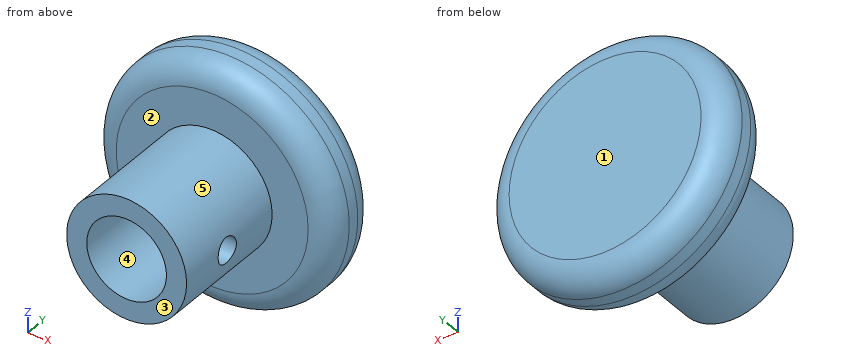
```python
from build123d import *

# Parameters (mm, degrees)
F0_R     = 6.35
F1_DEPTH = 19.05
F0_R_2   = 12.7
F2_DEPTH = 6.35
F4_D     = 8.4328
F4_DEPTH = 13.335
F4_TIP   = 2.5334687141
F6_R     = 2.54
F7_D     = 2.7051
F7_DEPTH = 7.62
F7_TIP   = 0.8126940303


with BuildPart() as f1:
    # F0 (on Front) → F1 (new body)
    with BuildSketch(Plane.XZ):
        Circle(F0_R)
    extrude(amount=F1_DEPTH)

    # F0 (on Front) → F2 (join)
    with BuildSketch(Plane.XZ):
        Circle(F0_R_2)
        Circle(F0_R, mode=Mode.SUBTRACT)
    extrude(amount=F2_DEPTH)

    # F4
    with Locations(Plane.XZ.offset(19.05)):
        with Locations((0, 0)):
            Hole(F4_D / 2, depth=F4_DEPTH)
            with Locations((0, 0, -(F4_DEPTH + F4_TIP / 2))):  # 118° drill point
                Cone(0, F4_D / 2, F4_TIP, mode=Mode.SUBTRACT)

    # F6
    f6_edges = [f1.edges().sort_by_distance(p)[0] for p in [
        (-12.7, -6.35, 0),
        (-12.7, 0, 0),
    ]]
    fillet(f6_edges, radius=F6_R)

    # F7 (one way)
    with BuildSketch(Plane(origin=(0, 0, 0), x_dir=(0, 1, 0), z_dir=(-1, 0, 0))):
        with Locations((-13.0086187273, 0)):
            Circle(F7_D / 2)
    extrude(amount=-F7_DEPTH, mode=Mode.SUBTRACT)
    with Locations(Plane(origin=(0, 0, 0), x_dir=(0, 1, 0), z_dir=(-1, 0, 0))):
        with Locations((-13.0086187273, 0)):
            with Locations((0, 0, -(F7_DEPTH + F7_TIP / 2))):  # 118° drill point
                Cone(0, F7_D / 2, F7_TIP, mode=Mode.SUBTRACT)


solid = f1.part
```
Could you check a few things on this model? Use its own coordinates, in mm. Face numbers are marked on the shaded views. A direction names the side the tool comes from. Round coordinates to 2 decimals unless told otherwise and drop trailing zeros. Write each loop counter-clockwise with the first axis right and the second up, starting at its lowest first coordinate (ties: lowest second). Pieces come first, ordered by that corner, then holes. Notation, with made-up numbers: M -33.75,55.5 L 20.25,55.5 A13 ccw 20.25,76.5 Z; hole C -3.5,22 d9. An arc over 180 degrees is marked long. Answer in a Markdown table with one row per item. Add a question column.
Q1. If we mould it in two halves opening along Z, with no side actions, what happens to the marked faces 3, 4 and 5? For each: +Z half, -Z half, draft (parallel to the pull), parting line (faces both ways), or undercut.
Q2. Imagine slicing it at A-A (y = -7.5). Please give me the cut outline in (x, z), then the cut area to 3 significant figures.
Q3. If I drill on line 1 (Z direction, x = 0, y = -11); line 2 (Z direction, x = 1.5, y = -13.5); line 3 (Y direction, x = 3, z = 7.25), over which ranges is the centre line in solid material (lowest first)? Write a range as from..to.
Q4. Will these pins go through, and if not, where does the flat tip stop? pin 1 Ø10 at (x, y) = (5, -12) entering from +Z; pin 2 Ø1 at (x, z) = (-7.5, 8.5) entering from +Y; pin 3 Ø11 at (x, z) = (0, 0) entering from +Y; pin 4 Ø8 at (x, z) = (10, 5) entering from -Y.
Q5. Imagine slicing it at B-B (y = -1.25). Please give me the cut outline in (x, z), then the cut area to 3 significant figures.
Q6. On a 3-axis mill with a long thin cutter (end or side, diameter ignored), from which of +Z, -Z, +X, -X, +Y, -Y can I reach the whole of each face in a straight line? I mean the marked faces 1 and 2. Say none if no direction works.
Values:
| question | item | result |
|---|---|---|
| 1 | face 3 | draft |
| 1 | face 4 | undercut |
| 1 | face 5 | parting line |
| 2 | outline | C 0,0 d12.7; hole C 0,0 d8.43 |
| 2 | area | 70.8 mm^2 |
| 3 | line 1 | -6.35..-4.22, 4.22..6.35 |
| 3 | line 2 | -6.17..-3.94, 3.94..6.17 |
| 3 | line 3 | -6.35..0 |
| 4 | pin 1 | z = 6.35 |
| 4 | pin 2 | y = -0.09 |
| 4 | pin 3 | y = 0 |
| 4 | pin 4 | y = -6.35 |
| 5 | outline | C 0,0 d24.7 |
| 5 | area | 479 mm^2 |
| 6 | face 1 | +Z, -Z, +X, -X, +Y |
| 6 | face 2 | -Y |
